Source: CAD feature listing. Evaluate the final solid. Frame: model axes, mm. Coordinates: 2 decimals unless noted, no trailing zeros. Write each loop counter-clockwise with the first axis right and the second up, starting at its lowest first coordinate (ties: lowest second). Pieces come first, ordered by that corner, then holes. Notation, with made-up numbers: (88.5, 3) - (147.5, 3) arc R21 ccw to (147.5, 14) - close; hole circle Ø11 at (65.5, 10.5). An arc over 180 degrees is marked (long way). One line per question, with ' | ' between items. Start each with the question number.
Q1. Cut plane A-A, the plane x = 0. Return loops of the section in (y, z).
Q2. Cut plane C-C, the plane x = 142. Return loops of the section in (y, z).
Q3. Line query: line 1 (X direction, y = 4.5, z = -10.25); line 2 (X direction, y = 124, z = 1.75); line 3 (Y direction, x = 26, z = 2.75). Output: solid intervals per line, ascending.
Q4. Contact query for flat-ended pins moving along their axis: P1, Ø2.5, axis at y = 72.5, z = 1.5, coming from the -X side; P2, Ø2.5, axis at y = -106.5, z = 0.5, coming from the -X side; P3, Ø8, axis at x = 70, z = 5, coming from the +Y side. Output: stop coordinate, or through.
Q5. Cut plane D-D, the plane y = -111.5. Return loops of the section in (x, z), plus the area to 3 significant figures.
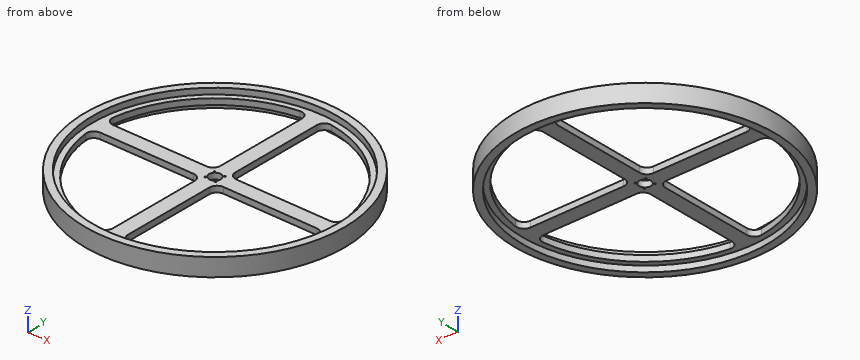
Autodesk Inventor part; units mm, degrees
ref_plane "Work Plane1" through (0, 0, 0) normal (0, 0, 1) x (1, 0, 0)
ref_plane "YZ Plane" through (0, 0, 0) normal (1, 0, 0) x (0, 1, 0)
ref_plane "XZ Plane" through (0, 0, 0) normal (0, 1, 0) x (-1, 0, 0)
sketch "Sketch1" plane through (0, 0, 0) normal (0, 0, 1) x (1, 0, 0)
  circle A0 centre (0, 0) radius 175
  dimension "d0" = 350
extrude "Extrusion1" add sketch "Sketch1" along normal mid plane 24
sketch "Sketch2" plane through (0, 0, 12) normal (0, 0, 1) x (1, 0, 0)
  circle A0 centre (0, 0) radius 165
  dimension "d3" = 330
extrude "Extrusion2" cut sketch "Sketch2" against normal blind 8
ref_plane "Work Plane1" through (0, 0, 0) normal (0, 0, 1) x (1, 0, 0)
mirror "Mirror1" about plane through (0, 0, 0) normal (0, 0, 1) of "Extrusion2"
sketch "Sketch3" plane through (0, 0, 4) normal (0, 0, 1) x (1, 0, 0)
  circle A0 centre (0, 0) radius 8
  line L0 (-10, -10) -> (-10, -157.1822)
  line L1 (10, -10) -> (10, -157.1822)
  line L2 (0, 0) -> (0, -162.7163) construction
  arc A1 (-157.1822, -10) -> (-10, -157.1822) centre (0, 0) ccw
  line L3 (-10, -10) -> (-157.1822, -10)
  arc A2 (10, -157.1822) -> (157.1822, -10) centre (0, 0) ccw
  line L4 (10, -10) -> (157.1822, -10)
  dimension "d7" = 16
  dimension "d8" = 20
  dimension "d9" = 157.5
  dimension "d10" = 10
extrude "Extrusion3" cut sketch "Sketch3" against normal blind 8 contours L0 A1 L3 | L4 A2 L1
pattern_circular "Circular Pattern1" count 2 over 360 about axis through (0, 0, 12) along (0, 0, -1) of "Extrusion3"
fillet "Fillet1" radius 10 12 edges at (-10, 157.1822, 0) (-157.1822, 10, 0) (-10, 10, 0) (-10, -10, 0) (-157.1822, -10, 0) (-10, -157.1822, 0) (10, -157.1822, 0) (10, -10, 0) (157.1822, -10, 0) (157.1822, 10, 0) (10, 10, 0) (10, 157.1822, 0)
extrude "Extrusion4" cut sketch "Sketch3" against normal up to surface (8 mm away) contours A0
sketch "Sketch4" plane through (0, 0, 4) normal (0, 0, 1) x (1, 0, 0)
  circle A0 centre (0, 0) radius 8
  circle A1 centre (0, 0) radius 10 construction
  line L0 (0, 0) -> (-7.0711, 7.0711) construction
  line L1 (0, 0) -> (0, 20.2635) construction
  dimension "d21" = 20
  dimension "d22" = 45
hole "Hole1" at (-7.0711, 7.0711, 4) direction (0, 0, -1) diameter 2 depth 8
pattern_circular "Circular Pattern2" count 4 over 360 about axis through (0, 0, 4) along (0, 0, -1) of "Hole1"
properties part number "05"
Reply:
1) outline: (-175, -12) - (-165, -12) - (-165, -4) - (-8, -4) - (-8, 4) - (-165, 4) - (-165, 12) - (-175, 12) - close; (8, -4) - (165, -4) - (165, -12) - (175, -12) - (175, 12) - (165, 12) - (165, 4) - (8, 4) - close
2) outline: (-102.28, -12) - (-84.03, -12) - (-84.03, -4) - (-68.13, -4) - (-68.13, 4) - (-84.03, 4) - (-84.03, 12) - (-102.28, 12) - close; (-10, -4) - (10, -4) - (10, 4) - (-10, 4) - close; (68.13, -4) - (84.03, -4) - (84.03, -12) - (102.28, -12) - (102.28, 12) - (84.03, 12) - (84.03, 4) - (68.13, 4) - close
3) line 1: x = -174.94 to -164.94, 164.94 to 174.94 | line 2: x = -123.49 to -97.11, -10 to 10, 97.11 to 123.49 | line 3: y = -173.06 to -155.34, -10 to 10, 155.34 to 173.06
4) P1: stops at x = -159.84 | P2: stops at x = -139.81 | P3: stops at y = 162.08
5) outline: (-134.88, -12) - (-121.63, -12) - (-121.63, -4) - (-111.24, -4) - (-111.24, 4) - (-121.63, 4) - (-121.63, 12) - (-134.88, 12) - close; (-10, -4) - (10, -4) - (10, 4) - (-10, 4) - close; (111.24, -4) - (121.63, -4) - (121.63, -12) - (134.88, -12) - (134.88, 12) - (121.63, 12) - (121.63, 4) - (111.24, 4) - close | area: 962 mm^2
